from build123d import *

# Parameters (mm, degrees)
SKETCH1_R               = 15.875
BOSS_EXTRUDE1_DEPTH     = 25.4
CUT_EXTRUDE1_DEPTH      = 34.89972345
CUT_EXTRUDE1_DEPTH_BACK = 34.89972345
SKETCH2_W               = 6.604
SKETCH2_H               = 13.97
SKETCH3_R               = 3.175
CUT_EXTRUDE2_DEPTH      = 12.7


with BuildPart() as part:
    # Sketch1 → Boss-Extrude1 (new body)
    with BuildSketch(Plane(origin=(0, 0, 0), x_dir=(1, 0, 0), z_dir=(0, 1, 0))):
        with Locations(Location((0, 0, 0), (0, 0, 270))):
            Circle(SKETCH1_R)
    extrude(amount=BOSS_EXTRUDE1_DEPTH)

    # Sketch2 → Cut-Extrude1 (cut, two sides: drawn at the far end of the back side and taken through both)
    with BuildSketch(Plane(origin=(0, 0, 0), x_dir=(0, 0, -1), z_dir=(1, 0, 0)).offset(-CUT_EXTRUDE1_DEPTH_BACK)):
        with Locations((12.573, 6.985)):
            Rectangle(SKETCH2_W, SKETCH2_H)
        with Locations((-12.573, 6.985)):
            Rectangle(SKETCH2_W, SKETCH2_H)
    extrude(amount=CUT_EXTRUDE1_DEPTH + CUT_EXTRUDE1_DEPTH_BACK, mode=Mode.SUBTRACT)

    # Sketch3 → Cut-Extrude2 (cut)
    with BuildSketch(Plane(origin=(0, 25.4, 0), x_dir=(1, 0, 0), z_dir=(0, 1, 0))):
        with Locations(Location((0, 0, 0), (0, 0, 270))):
            Circle(SKETCH3_R)
    extrude(amount=-CUT_EXTRUDE2_DEPTH, mode=Mode.SUBTRACT)


solid = part.part
CAD build for the part. Positions are in the model's coordinates, mm. A direction names the side the tool comes from. Give positions to 0.01 mm unless a question says otherwise; leave off trailing zeros. Loops run counter-clockwise (first coordinate to the right, second up) from the corner with the lowest first, then second, coordinate; pieces in that order, holes last. Notation, with made-up numbers: M -30,-2 L -19,-2 A11 ccw -19,9 Z; hole C -4,33.5 d1. An arc over 180 degrees is marked long. One line per question, with ' | ' between items. Start each with the question number.
1. Saw through at A-A on z = 0. Give the cut face in (x, y) (3 decimals), plus the area to 3 significant figures.
2. Saw through at B-B on x = 0. Give the cut face in (y, z) (3 decimals), plus the area to 3 significant figures.
3. Probe L1, parallel to X at y = 21.5, z = 0 (3 decimals); L2, parallel to Y at x = 4, z = 13; L3, parallel to Z at x = -12, y = 8.25. List the from-to ranges inside material, lowest first. Write a range as from..to.
4. 3-axis set-ups, long thin cutter, end or side, ignore diameter. For faces 5 (the face through (0, 7, -9.271)), 6 (the face through (0, 0, 0)), 7 (the face through (0, 7, 9.271)): which of +Z, -Z, +X, -X, +Y, -Y reach the whole face in a straight line?
5. Two-plate mould, pull along X, no slides. Class faces 1 (the face through (-6.08, 15.344, 14.664)), 2 (the face through (0, 12.7, 0)), 3 (the face through (0, 13.97, -12)), 4 (the face through (-1.93, 19.14, -2.52)): pulls with the +X half, pulls with the -X half, needs draft (parallel to the pull), parting line crosses it, or undercut.
6. Flat gauge pins, fed straight in: pin 1 (8 mm diameter, centred on x = 0.5, y = 7.5, fed in from +Z); pin 2 (1.5 mm diameter, centred on x = -9.5, y = 15, fed in from -Z); pin 3 (5.5 mm diameter, centred on x = -0.5, z = 13.5, fed in from -Y); pin 4 (2 mm diameter, centred on y = 12.5, z = -12.5, fed in from -X). Where does each tip first touch, or does it go through?
7. Saw through at C-C on y = 20. Give the cut face in (x, z) (3 decimals), plus the area to 3 significant figures.
8. Saw through at D-D on y = 9. Give the cut face in (x, z) (3 decimals), plus the area to 3 significant figures.
Result sheet:
1) outline: M -15.875,0 L 15.875,0 L 15.875,25.4 L 3.175,25.4 L 3.175,12.7 L -3.175,12.7 L -3.175,25.4 L -15.875,25.4 Z | area: 726 mm^2
2) outline: M 0,-9.271 L 13.97,-9.271 L 13.97,-15.875 L 25.4,-15.875 L 25.4,-3.175 L 12.7,-3.175 L 12.7,3.175 L 25.4,3.175 L 25.4,15.875 L 13.97,15.875 L 13.97,9.271 L 0,9.271 Z | area: 541 mm^2
3) L1: x = -15.875..-3.175, 3.175..15.875 | L2: y = 13.97..25.4 | L3: z = -9.27..9.27
4) face 5: -Z, +X, -X, -Y | face 6: +Z, -Z, +X, -X, -Y | face 7: +Z, +X, -X, -Y
5) face 1: parting line crosses it | face 2: undercut | face 3: needs draft | face 4: undercut
6) pin 1: stops at z = 9.27 | pin 2: stops at z = -13.25 | pin 3: stops at y = 13.97 | pin 4: passes through
7) outline: C 0,0 d31.75; hole C 0,0 d6.35 | area: 760 mm^2
8) outline: M -12.887,-9.271 L 12.887,-9.271 A15.875 ccw 12.887,9.271 L -12.887,9.271 A15.875 ccw Z | area: 553 mm^2
